Part model, mm, in its own coordinate system. Coordinates: 2 decimals unless noted, no trailing zeros. Write each loop counter-clockwise with the first axis right and the second up, starting at its lowest first coordinate (ties: lowest second). Pieces come first, ordered by that corner, then holes. Notation, with made-up numbers: (71.25, 82.5) - (103.25, 82.5) arc R29 ccw to (103.25, 114.5) - close; hole circle Ø7 at (16.25, -18). An arc over 180 degrees is marked (long way). Write each question's results on one line, items separated by ' | '.
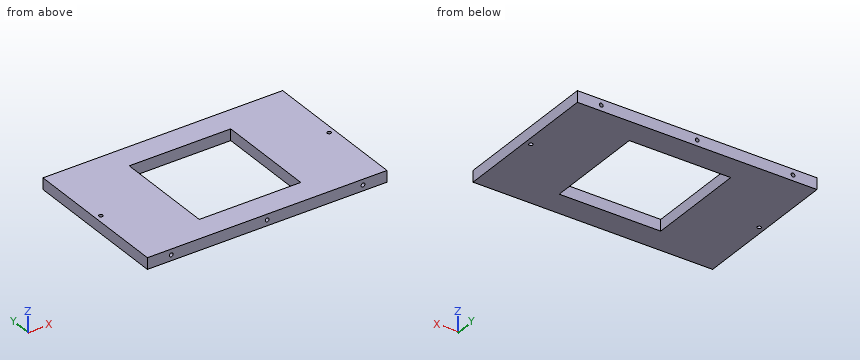
Autodesk Inventor part; units mm, degrees
ref_plane "YZ Plane" through (0, 0, 0) normal (1, 0, 0) x (0, 1, 0)
ref_plane "XZ Plane" through (0, 0, 0) normal (0, 1, 0) x (-1, 0, 0)
ref_plane "XY Plane" through (0, 0, 0) normal (0, 0, 1) x (1, 0, 0)
sketch "Sketch1" plane through (0, 0, 0) normal (0, 0, 1) x (1, 0, 0)
  line L0 (0, 0) -> (190, 0)
  line L1 (190, 0) -> (190, 120)
  line L2 (190, 120) -> (0, 120)
  line L3 (0, 120) -> (0, 0)
  dimension "d0" = 190
  dimension "d1" = 120
extrude "Extrusion1" add sketch "Sketch1" along normal blind 9
sketch "Sketch2" plane through (0, 0, 9) normal (0, 0, 1) x (1, 0, 0)
  line L0 (190, 0) -> (190, 120)
  line L1 (190, 120) -> (0, 120)
  line L2 (0, 120) -> (0, 0)
  line L3 (0, 0) -> (190, 0)
  line L4 (135.25, 19.75) -> (54.75, 19.75)
  line L5 (54.75, 19.75) -> (54.75, 100.25)
  line L6 (54.75, 100.25) -> (135.25, 100.25)
  line L7 (135.25, 100.25) -> (135.25, 19.75)
  line L8 (135.25, 19.75) -> (54.75, 100.25) construction
  line L9 (54.75, 19.75) -> (135.25, 100.25) construction
  point P0 (95, 60)
  dimension "d4" = 80.5
  dimension "d5" = 80.5
extrude "Extrusion2" cut sketch "Sketch2" against normal blind 10 contours L4 L5 L6 L7
sketch "Sketch3" plane through (0, 120, 0) normal (0, 1, 0) x (1, 0, 0)
  line L0 (190, 0) -> (0, 0)
  line L1 (0, 0) -> (0, -9)
  line L2 (190, -9) -> (0, -9)
  line L3 (190, 0) -> (190, -9)
  circle A0 centre (19, -4.5) radius 1.5
  circle A1 centre (95, -4.5) radius 1.5
  circle A2 centre (171, -4.5) radius 1.5
  point P0 (0, 0)
  dimension "d8" = 3
  dimension "d9" = 3
  dimension "d10" = 3
extrude "Extrusion3" cut sketch "Sketch3" against normal blind 10 contours A0 | A1 | A2
sketch "Sketch4" plane through (0, 0, 0) normal (0, -1, 0) x (1, 0, 0)
  circle A0 centre (19, 4.5) radius 1.5
  circle A1 centre (95, 4.5) radius 1.5
  circle A2 centre (171, 4.5) radius 1.5
  point P0 (0, 0)
extrude "Extrusion4" cut sketch "Sketch4" against normal blind 10
sketch "Sketch5" plane through (0, 0, 9) normal (0, 0, 1) x (1, 0, 0)
  line L0 (190, 120) -> (0, 120)
  line L1 (0, 0) -> (190, 0)
  line L2 (0, 120) -> (9, 120)
  line L3 (9, 120) -> (9, 0)
  line L4 (9, 0) -> (0, 0)
  line L5 (0, 0) -> (0, 120)
  line L6 (190, 120) -> (181, 120)
  line L7 (181, 120) -> (181, 0)
  line L8 (181, 0) -> (190, 0)
  line L9 (190, 0) -> (190, 120)
  circle A0 centre (4.5, 60) radius 1.5
  circle A1 centre (185.5, 60) radius 1.5
  dimension "d15" = 9
  dimension "d16" = 9
  dimension "d17" = 3
  dimension "d18" = 3
extrude "Extrusion5" cut sketch "Sketch5" against normal blind 10 contours A0 | A1
properties part number "Lateral1-2_3DPrint"
(1) Wall check: line 1 (X direction, y = 116, z = 4.5); line 2 (Y direction, x = 121.5, z = 0.75); line 3 (Z direction, x = 19, y = 6). Give the ranges that are in metal, low to high. Write a range as from..to.
Return value:
line 1: x = 0..17.5, 20.5..93.5, 96.5..169.5, 172.5..190 | line 2: y = 0..19.75, 100.25..120 | line 3: z = 0..3, 6..9
(2) Flat gauge pins, fed straight in: P1, Ø4, axis at x = 19, z = 4.5, coming from the +Y side; P2, Ø2.5, axis at x = 95, z = 4.5, coming from the -Y side; P3, Ø2.5, axis at x = 185.5, y = 60, coming from the +Z side; P4, Ø1.8, axis at x = 95, z = 4.5, coming from the +Y side. Where does each tip first touch, or does it go through?
Return value:
P1: stops at y = 120 | P2: stops at y = 10 | P3: passes through | P4: stops at y = 110
(3) Saw through at B-B on z = 4.5. Count the separate pieces of the cut face and the enclosed holes in it, then the cut area to 3 significant figures.
Return value:
separate pieces: 1 | enclosed holes: 3 | area: 16,100 mm^2
(4) Saw through at A-A on y = 36. Write the cut outline in (x, z), then the cut area to 4 significant figures.
Return value:
outline: (0, 0) - (54.75, 0) - (54.75, 9) - (0, 9) - close; (135.25, 0) - (190, 0) - (190, 9) - (135.25, 9) - close | area: 985.5 mm^2
